```python
from build123d import *

# Parameters (mm, degrees)
CROQUIS2_W              = 500
CROQUIS2_H              = 720
SALIENTE_EXTRUIR1_DEPTH = 30
CROQUIS3_W              = 440
CROQUIS3_H              = 520.616152256
CORTAR_EXTRUIR1_DEPTH   = 440.31765273
REDONDEO1_R             = 10
REDONDEO2_R             = 10
CROQUIS4_W              = 440
CROQUIS4_H              = 90
CORTAR_EXTRUIR4_DEPTH   = 5
CROQUIS9_W              = 480
CROQUIS9_H              = 20
CORTAR_EXTRUIR6_DEPTH   = 7
CROQUIS10_W             = 10
CROQUIS10_H             = 130
CORTAR_EXTRUIR7_DEPTH   = 20


with BuildPart() as part:
    # Croquis2 → Saliente-Extruir1 (new body)
    with BuildSketch(Plane.XY):
        Rectangle(CROQUIS2_W, CROQUIS2_H)
    extrude(amount=SALIENTE_EXTRUIR1_DEPTH)

    # Croquis3 → Cortar-Extruir1 (cut, through all)
    with BuildSketch(Plane(origin=(0, 0, 0), x_dir=(-1, 0, 0), z_dir=(0, 0, -1))):
        with Locations((0, -50.308076128)):
            Rectangle(CROQUIS3_W, CROQUIS3_H)
    extrude(amount=-CORTAR_EXTRUIR1_DEPTH, mode=Mode.SUBTRACT)

    # Redondeo1
    redondeo1_edges = [part.edges().sort_by_distance(p)[0] for p in [
        (0, -360, 0),
    ]]
    fillet(redondeo1_edges, radius=REDONDEO1_R)

    # Redondeo2
    redondeo2_edges = [part.edges().sort_by_distance(p)[0] for p in [
        (0, -360, 30),
    ]]
    fillet(redondeo2_edges, radius=REDONDEO2_R)

    # Croquis4 → Cortar-Extruir4 (cut)
    with BuildSketch(Plane(origin=(0, 0, 0), x_dir=(-1, 0, 0), z_dir=(0, 0, -1))):
        with Locations((0, 284.028138346)):
            Rectangle(CROQUIS4_W, CROQUIS4_H)
    extrude(amount=-CORTAR_EXTRUIR4_DEPTH, mode=Mode.SUBTRACT)

    # Croquis9 → Cortar-Extruir6 (cut)
    with BuildSketch(Plane.XY.offset(30)):
        with Locations((10, 300)):
            Rectangle(CROQUIS9_W, CROQUIS9_H)
    extrude(amount=-CORTAR_EXTRUIR6_DEPTH, mode=Mode.SUBTRACT)

    # Croquis10 → Cortar-Extruir7 (cut)
    with BuildSketch(Plane(origin=(250, 0, 0), x_dir=(0, 0, -1), z_dir=(1, 0, 0))):
        with Locations((-25, 295)):
            Rectangle(CROQUIS10_W, CROQUIS10_H)
    extrude(amount=-CORTAR_EXTRUIR7_DEPTH, mode=Mode.SUBTRACT)


solid = part.part
```
Geometry: final body of the model. Coordinates: model frame, mm. A direction names the side the tool comes from. Round coordinates to 2 decimals unless told otherwise and drop trailing zeros. Order: outer loops, then holes, each group sorted by start corner. A loop starts at its lowest first (then second) coordinate and runs counter-clockwise, first axis right, second up. Notation, with made-up numbers: (-6, 17) -> (21, 17) arc R27 ccw to (21, 46) -> close; hole circle Ø8 at (-4, -31.5). An arc over 180 degrees is marked (long way). Use one line per item in the form item = value.
(1) Access query for faces 5 (the face through (-1, 217, 0)), 6 (the face through (240, 294, 20)), 7 (the face through (3, -310.616, 15)). Directions: +Z, -Z, +X, -X, +Y, -Y. A direction counts if a zero-diameter tool reaches every point of the face in a straight line with its end or side. Return the directions, or none.
Results list:
face_5 = -Z, +X, -X, +Y, -Y
face_6 = +Z, +X, +Y
face_7 = +Z, -Z
(2) Ray query, probe 1 along Y at (x, z) = (-52.5, 18.5); probe 2 along X at (y, z) = (-235, 9.75); probe 3 along Y at (x, z) = (-145.5, 25.5). Return the intervals inside material, ascending. Write a range as [from, to].
Results list:
probe_1 = [-360, -310.62], [210, 360]
probe_2 = [-250, -220], [220, 250]
probe_3 = [-358.35, -310.62], [210, 290], [310, 360]
(3) Section C-C on y = 255. Return loops of the section in (x, z).
Results list:
outline = (-250, 0) -> (-220, 0) -> (-220, 5) -> (220, 5) -> (220, 0) -> (250, 0) -> (250, 20) -> (230, 20) -> (230, 30) -> (-250, 30) -> close
(4) First-contact query: pin 1 Ø10 at (x, y) = (236.5, 294.5) entering from +Z; pin 2 Ø3.5 at (x, z) = (-20, 28) entering from -Y; pin 3 Ø3 at (x, z) = (-45.5, 7.5) entering from -Y. Flat tips, straight axial feed; report the tip coordinate or a pass-through.
Results list:
pin_1 = 20
pin_2 = -357.81
pin_3 = -359.95
(5) Section B-B on y = 83. Return loops of the section in (x, z).
Results list:
outline = (-250, 0) -> (-220, 0) -> (-220, 30) -> (-250, 30) -> close; (220, 0) -> (250, 0) -> (250, 30) -> (220, 30) -> close
(6) Draft query along X for faces 1 (the face through (3, 285, 5)), 2 (the face through (-3, 300, 23)), 3 (the face through (-220, -54, 15)), 4 (the face through (-250, -5, 15)). Return one class per face: pulls with the +X half, pulls with the -X half, needs draft (parallel to the pull), parting line crosses it, or undercut.
Results list:
face_1 = undercut
face_2 = needs draft
face_3 = undercut
face_4 = pulls with the -X half
(7) Section A-A on x = 176.5. Return loops of the section in (y, z).
Results list:
outline = (-360, 10) arc R10 ccw to (-350, 0) -> (-310.62, 0) -> (-310.62, 30) -> (-350, 30) arc R10 ccw to (-360, 20) -> close; (210, 0) -> (239.03, 0) -> (239.03, 5) -> (329.03, 5) -> (329.03, 0) -> (360, 0) -> (360, 30) -> (310, 30) -> (310, 23) -> (290, 23) -> (290, 30) -> (210, 30) -> close
